Answer from the drawing. Dimensions are ordinates in mm from the lowest x, y and z of the part. A direction names the side the tool comes from. Coordinates: 2 decimals unless noted, no trailing zeros. Write each loop counter-clockwise with the first axis right and the second up, starting at its lowest first coordinate (ties: lowest second). Pieces come first, ordered by that corner, then holes. Notation, with made-up numbers: (-24.5, 35) -> (10.5, 35) arc R6 ccw to (10.5, 40) -> close; hole circle Ø4 at (71, 22.5). An arc over 180 degrees is marked (long way). One line per item, written item: value. Start each with the question number.
1. For the marked faces 5, 6 and 7, determine the directions among +Z, -Z, +X, -X, +Y, -Y from which every point of the face is accessible in a straight line to the end or side of a thin tool.
2. Given P1, Ø3, axis at y = 73, z = 11, coming from the -X side, flat-ended and moving along its own axis, determine where the tip first touches the part or whether it passes through.
3. Find section B-B, the plane y = 50.5. Write down the section's boundary in (x, z), and give its area (3 significant figures).
4. Consider line 1 along Z through (x, y) = (43, 4.5). Determine where the line is inside the solid, lowest interval first.
5. Find section A-A, the plane x = 91. Write down the section's boundary in (y, z).
6. For a pull along Z with two mould halves and no side action, classify the marked faces 1, 2, 3 and 4 as pulls with the +Z half, pulls with the -Z half, needs draft (parallel to the pull), parting line crosses it, or undercut.
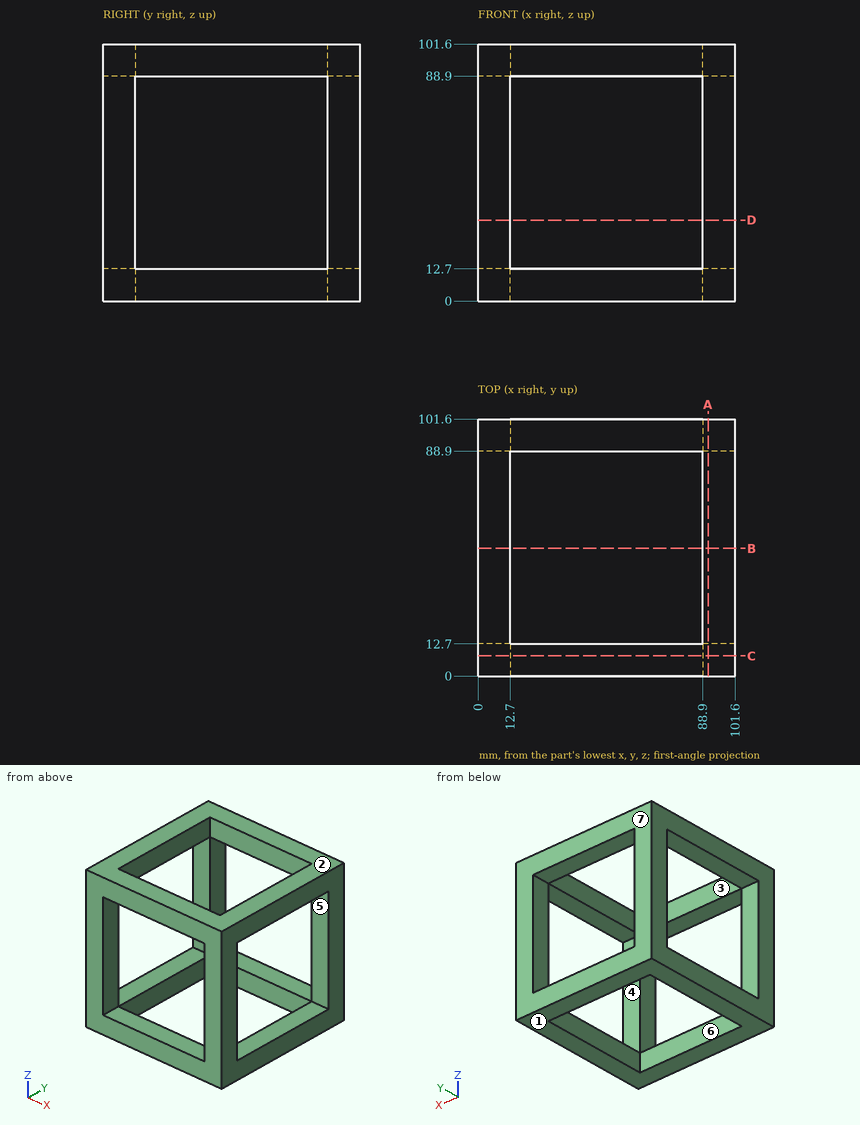
Answer block:
1. face 5: +X, -X
1. face 6: +Z, -Z
1. face 7: +Z, -Z, +X, -X, +Y
2. P1: stops at x = 0
3. outline: (0, 0) -> (12.7, 0) -> (12.7, 12.7) -> (0, 12.7) -> close; (0, 88.9) -> (12.7, 88.9) -> (12.7, 101.6) -> (0, 101.6) -> close; (88.9, 0) -> (101.6, 0) -> (101.6, 12.7) -> (88.9, 12.7) -> close; (88.9, 88.9) -> (101.6, 88.9) -> (101.6, 101.6) -> (88.9, 101.6) -> close
3. area: 645 mm2
4. line 1: z = 0 to 12.7, 88.9 to 101.6
5. outline: (0, 0) -> (101.6, 0) -> (101.6, 101.6) -> (0, 101.6) -> close; hole (12.7, 12.7) -> (88.9, 12.7) -> (88.9, 88.9) -> (12.7, 88.9) -> close
6. face 1: pulls with the -Z half
6. face 2: pulls with the +Z half
6. face 3: needs draft
6. face 4: undercut
